```python
from build123d import *

# Parameters (mm, degrees)
SKETCH1_R           = 1.25
BOSS_EXTRUDE1_DEPTH = 3


with BuildPart() as part:
    # Sketch1 → Boss-Extrude1 (new body)
    with BuildSketch(Plane(origin=(0, 0, 0), x_dir=(1, 0, 0), z_dir=(0, 1, 0))):
        with BuildLine():
            ThreePointArc((0.75263713, 8.414705215), (-8.448297255, 0), (0.75263713, -8.414705215))
            ThreePointArc((0.75263713, -8.414705215), (1.926901999, -8.002285906), (2.941567446, -7.281562869))
            Line((2.941567446, -7.281562869), (7.281562869, -2.941567446))
            ThreePointArc((7.281562869, -2.941567446), (8.5, 0), (7.281562869, 2.941567446))
            Line((7.281562869, 2.941567446), (2.941567446, 7.281562869))
            ThreePointArc((2.941567446, 7.281562869), (1.926901999, 8.002285906), (0.75263713, 8.414705215))
        make_face()
        Circle(SKETCH1_R, mode=Mode.SUBTRACT)
    extrude(amount=BOSS_EXTRUDE1_DEPTH)


solid = part.part
```
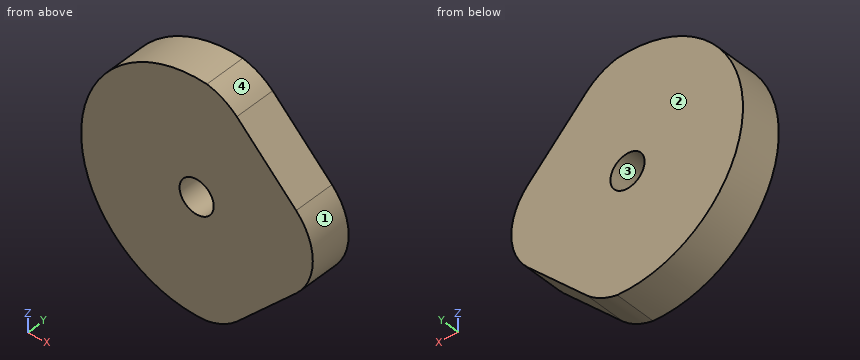
Geometry check sheet. Reference: the model listing, model coordinates, mm. Face numbers are marked on the shaded views. Round coordinates to 2 decimals unless told otherwise and drop trailing zeros. Loops run counter-clockwise (first coordinate to the right, second up) from the corner with the lowest first, then second, coordinate; pieces in that order, holes last. Notation, with made-up numbers: M 1,-5.75 L 46,-5.75 A17 cw 46,27.25 Z; hole C -20,81 d3. An arc over 180 degrees is marked long. Return JSON: item names as keys, results as strings. Group by question number.
(1) Scan lines: line 1 along Z through (x, y) = (0, 1.45); line 2 along X through (y, z) = (1.85, 0); line 3 along X through (y, z) = (2.3, 0.5). Record each from-to range of solid material in increasing order. Write a range as [from, to].
(2) Section check A-A, the plane x = 0. Enter the section's corners in (y, z), and give its area (3 significant figures).
(3) Section check C-C, the plane y = 1.5. Enter the section's corners in (x, z), and give its area (3 significant figures).
(4) Go/stop test with flat-tipped pins: pin 1 (1.5 mm diameter, centred on y = 0.5, z = 6, fed in from +X); pin 2 (1 mm diameter, centred on x = 2.5, y = 1, fed in from +Z). Record where each tip stops, or that it passes through.
(5) Section check D-D, the plane z = -2.25. Enter the section's corners in (x, y), and give its area (3 significant figures).
(6) Section check B-B, the plane z = 0. Enter the section's corners in (x, y).
(7) Mould release check, pull along Z, two halves, no side actions. Record for the marked faces 1, 2, 3 and 4: pulls with the +Z half, pulls with the -Z half, needs draft (parallel to the pull), parting line crosses it, or undercut.
Data:
{
 "1": {"line 1": "[-8.45, -1.25], [1.25, 8.45]", "line 2": "[-8.45, -1.25], [1.25, 8.5]", "line 3": "[-8.43, -1.15], [1.15, 8.47]"},
 "2": {"outline": "M 0,-8.45 L 3,-8.45 L 3,-1.25 L 0,-1.25 Z; M 0,1.25 L 3,1.25 L 3,8.45 L 0,8.45 Z", "area": "43.2 mm²"},
 "3": {"outline": "M 0.75,-8.41 A4.46 ccw 2.94,-7.28 L 7.28,-2.94 A4.16 ccw 7.28,2.94 L 2.94,7.28 A4.46 ccw 0.75,8.41 A8.45 ccw long Z; hole C 0,0 d2.5", "area": "204 mm²"},
 "4": {"pin 1": "x = 4.97", "pin 2": "z = 7.96"},
 "5": {"outline": "M -8.14,0 L 7.84,0 L 7.84,3 L -8.14,3 Z", "area": "47.9 mm²"},
 "6": {"outline": "M -8.45,0 L -1.25,0 L -1.25,3 L -8.45,3 Z; M 1.25,0 L 8.5,0 L 8.5,3 L 1.25,3 Z"},
 "7": {"face 1": "parting line crosses it", "face 2": "needs draft", "face 3": "undercut", "face 4": "pulls with the +Z half"}
}
